Geometry: final body of the model. Coordinates: model frame, mm. A direction names the side the tool comes from. Coordinates: 2 decimals unless noted, no trailing zeros. Order: outer loops, then holes, each group sorted by start corner. A loop starts at its lowest first (then second) coordinate and runs counter-clockwise, first axis right, second up. Notation, with made-up numbers: (4, -40) - (33, -40) arc R15 cw to (33, -25) - close; hole circle Ø5 at (-26.75, 48). An arc over 180 degrees is marked (long way). Use a Markdown table: item, result. Add a question column.
```python
from build123d import *

# Parameters (mm, degrees)
SKETCH1_W           = 13
SKETCH1_H           = 17
BOSS_EXTRUDE1_DEPTH = 30
SKETCH2_R           = 5.75
CUT_EXTRUDE1_DEPTH  = 5
SKETCH3_W           = 3
SKETCH3_H           = 10
CUT_EXTRUDE2_DEPTH  = 32.851216617
SKETCH4_W           = 27
SKETCH4_H           = 17
BOSS_EXTRUDE2_DEPTH = 2
SKETCH5_W           = 7
SKETCH5_H           = 17
BOSS_EXTRUDE3_DEPTH = 20
SKETCH6_W           = 7
SKETCH6_H           = 3.5
BOSS_EXTRUDE4_DEPTH = 5
SKETCH7_R           = 2.5
CUT_EXTRUDE3_DEPTH  = 7
CUT_EXTRUDE4_DEPTH  = 42.632319176
CUT_EXTRUDE5_DEPTH  = 1
SKETCH11_W          = 0.75
SKETCH11_H          = 24
CUT_EXTRUDE6_DEPTH  = 1
SKETCH12_W          = 8
SKETCH12_H          = 0.75
CUT_EXTRUDE7_DEPTH  = 1
CUT_EXTRUDE8_DEPTH  = 13
SKETCH14_W          = 10
SKETCH14_H          = 15
CUT_EXTRUDE9_DEPTH  = 3
CHAMFER1_SIZE       = 3
BOSS_EXTRUDE5_DEPTH = 8
BOSS_EXTRUDE6_DEPTH = 1


with BuildPart() as part:
    # Sketch1 → Boss-Extrude1 (new body)
    with BuildSketch(Plane(origin=(0, 0, 0), x_dir=(1, 0, 0), z_dir=(0, 1, 0))):
        Rectangle(SKETCH1_W, SKETCH1_H)
    extrude(amount=BOSS_EXTRUDE1_DEPTH)

    # Sketch2 → Cut-Extrude1 (cut)
    with BuildSketch(Plane.ZY.offset(6.5)):
        with Locations((0, -2)):
            Circle(SKETCH2_R)
    extrude(amount=-CUT_EXTRUDE1_DEPTH, mode=Mode.SUBTRACT)

    # Sketch3 → Cut-Extrude2 (cut, through all)
    with BuildSketch(Plane.XZ):
        with Locations((5, 0)):
            Rectangle(SKETCH3_W, SKETCH3_H)
    extrude(amount=-CUT_EXTRUDE2_DEPTH, mode=Mode.SUBTRACT)

    # Sketch4 → Boss-Extrude2 (add)
    with BuildSketch(Plane(origin=(0, 30, 0), x_dir=(1, 0, 0), z_dir=(0, 1, 0))):
        with Locations((7, 0)):
            Rectangle(SKETCH4_W, SKETCH4_H)
    extrude(amount=BOSS_EXTRUDE2_DEPTH)

    # Sketch5 → Boss-Extrude3 (add)
    with BuildSketch(Plane.XZ.offset(-30)):
        with Locations((17, 0)):
            Rectangle(SKETCH5_W, SKETCH5_H)
    extrude(amount=BOSS_EXTRUDE3_DEPTH)

    # Sketch6 → Boss-Extrude4 (add)
    with BuildSketch(Plane.XZ.offset(-30)):
        with Locations((10, 6.75)):
            Rectangle(SKETCH6_W, SKETCH6_H)
        with Locations((10, -6.75)):
            Rectangle(SKETCH6_W, SKETCH6_H)
    extrude(amount=BOSS_EXTRUDE4_DEPTH)

    # Sketch7 → Cut-Extrude3 (cut)
    with BuildSketch(Plane(origin=(20.5, 0, 0), x_dir=(0, 0, -1), z_dir=(1, 0, 0))):
        with Locations((0, 27.5)):
            Circle(SKETCH7_R)
    extrude(amount=-CUT_EXTRUDE3_DEPTH, mode=Mode.SUBTRACT)

    # Sketch9 → Cut-Extrude4 (cut, through all)
    with BuildSketch(Plane.XY.offset(8.5)):
        Polygon((0, 32), (-6.5, 16), (-6.5, 32), align=None)
    extrude(amount=-CUT_EXTRUDE4_DEPTH, mode=Mode.SUBTRACT)

    # Sketch10 → Cut-Extrude5 (cut)
    with BuildSketch(Plane.XZ):
        Polygon((-5.75, 5.390964663), (-5.75, 7.75), (6.5, 7.75), (6.5, 8.5), (-6.5, 8.5), (-6.5, 5.390964663), align=None)
        Polygon((-5.75, -7.75), (-5.75, -5.390964663), (-6.5, -5.390964663), (-6.5, -8.5), (6.5, -8.5), (6.5, -7.75), align=None)
    extrude(amount=-CUT_EXTRUDE5_DEPTH, mode=Mode.SUBTRACT)

    # Sketch11 → Cut-Extrude6 (cut)
    with BuildSketch(Plane(origin=(6.5, 0, 0), x_dir=(0, 0, -1), z_dir=(1, 0, 0))):
        with Locations((-8.125, 13)):
            Rectangle(SKETCH11_W, SKETCH11_H)
        with Locations((8.125, 13)):
            Rectangle(SKETCH11_W, SKETCH11_H)
    extrude(amount=-CUT_EXTRUDE6_DEPTH, mode=Mode.SUBTRACT)

    # Sketch12 → Cut-Extrude7 (cut)
    with BuildSketch(Plane.XZ.offset(-25)):
        with Locations((9.5, -8.125)):
            Rectangle(SKETCH12_W, SKETCH12_H)
        with Locations((9.5, 8.125)):
            Rectangle(SKETCH12_W, SKETCH12_H)
    extrude(amount=-CUT_EXTRUDE7_DEPTH, mode=Mode.SUBTRACT)

    # Sketch13 → Cut-Extrude8 (cut)
    with BuildSketch(Plane.XZ.offset(-10)):
        with BuildLine():
            Line((13.5, -8.5), (13.5, 8.5))
            add(Edge.make_bspline(
                [(13.5, -8.5), (15.857076701, -7.146482538), (17.987215619, 0.415145569), (16.168492061, 6.316191401), (13.5, 8.5)],
                knots=[0, 0, 0, 0, 0.5, 1, 1, 1, 1], degree=3))
        make_face()
    extrude(amount=-CUT_EXTRUDE8_DEPTH, mode=Mode.SUBTRACT)

    # Sketch14 → Cut-Extrude9 (cut)
    with BuildSketch(Plane(origin=(3.5, 0, 0), x_dir=(0, 0, -1), z_dir=(1, 0, 0))):
        with Locations((0, 22.5)):
            Rectangle(SKETCH14_W, SKETCH14_H)
    extrude(amount=-CUT_EXTRUDE9_DEPTH, mode=Mode.SUBTRACT)

    # Chamfer1
    chamfer1_edges = [part.edges().sort_by_distance(p)[0] for p in [
        (3.5, 15, 0),
    ]]
    chamfer(chamfer1_edges, length=CHAMFER1_SIZE - 0.0001)  # a hair under: the kernel refuses the full size

    # Sketch15 → Boss-Extrude5 (add)
    with BuildSketch(Plane.ZY.offset(6.5)):
        with BuildLine():
            Line((-7.322463691, 1), (-6.32455532, 1))
            ThreePointArc((-6.32455532, 1), (0, 5), (6.32455532, 1))
            Line((6.32455532, 1), (7.322463691, 1))
            ThreePointArc((7.322463691, 1), (0, 5.913183588), (-7.322463691, 1))
        make_face()
    extrude(amount=BOSS_EXTRUDE5_DEPTH)

    # Sketch16 → Boss-Extrude6 (add)
    with BuildSketch(Plane.ZY.offset(14.5)):
        with BuildLine():
            Line((-7.322463691, 1), (7.322463691, 1))
            ThreePointArc((7.322463691, 1), (0, 5.913183588), (-7.322463691, 1))
        make_face()
    extrude(amount=BOSS_EXTRUDE6_DEPTH)


solid = part.part
```
1) Section C-C (y = 5.5). Return loops of the section in (x, z), then the cut area to 3 significant figures.
2) Section B-B (y = 9). Return loops of the section in (x, z).
3) Set-up query: faces 1 (the face through (-5.75, 0.5, 6.6)), 2 (the face through (-1.5, 1, 0)), 3 (the face through (19, 10, 0)), 4 (the face through (-5.75, 0.5, -6.6)), 5 (the face through (0.5, 23, 0)). Return all of +Z, -Z, +X, -X, +Y, -Y with unobstructed straight access to the full face (end or side cutting, diameter ignored); none if empty.
4) Draft query along Z for faces 6 (the face through (2, 13.5, 0.1)), 7 (the face through (4, 17, -8.5)), 8 (the face through (20.5, 21, 0)). Return one class per face: pulls with the +Z half, pulls with the -Z half, needs draft (parallel to the pull), parting line crosses it, or undercut.
5) Section D-D (x = -7). Return loops of the section in (y, z).
6) Ray query, line 1 along Z through (x, y) = (11.5, 29); line 2 along Y through (x, z) = (16.25, 0); line 3 along Z through (x, y) = (15.25, 27.5). Return the intervals inside material, ascending.
7) Pin query (flat end, axial travel): pin 1 (4.5 mm diameter, centred on y = 11.5, z = 3, fed in from -X); pin 2 (0.8 mm diameter, centred on x = 10, z = -8.5, fed in from -Y); pin 3 (4.5 mm diameter, centred on y = 2.5, z = 1.5, fed in from +X). Return the tip coordinate at first contact, or that it passes through.
8) Section A-A (x = 9). Return loops of the section in (y, z).
Values follow:
| question | item | result |
|---|---|---|
| 1 | outline | (-15.5, -2.52) - (-6.5, -2.52) - (-6.5, -8.5) - (5.5, -8.5) - (5.5, -7.75) - (6.5, -7.75) - (6.5, -5) - (3.5, -5) - (3.5, 5) - (6.5, 5) - (6.5, 7.75) - (5.5, 7.75) - (5.5, 8.5) - (-6.5, 8.5) - (-6.5, 2.52) - (-15.5, 2.52) - close |
| 1 | area | 235 mm² |
| 2 | outline | (-6.5, -8.5) - (5.5, -8.5) - (5.5, -7.75) - (6.5, -7.75) - (6.5, -5) - (3.5, -5) - (3.5, 5) - (6.5, 5) - (6.5, 7.75) - (5.5, 7.75) - (5.5, 8.5) - (-6.5, 8.5) - close |
| 3 | face 1 | +Z, -X, -Y |
| 3 | face 2 | -Y |
| 3 | face 3 | +Z, -Z, +X, -Y |
| 3 | face 4 | -Z, -X, -Y |
| 3 | face 5 | none |
| 4 | face 6 | undercut |
| 4 | face 7 | pulls with the -Z half |
| 4 | face 8 | needs draft |
| 5 | outline | (1, -7.32) arc R7.91 ccw to (1, 7.32) - (1, 6.32) arc R7 cw to (1, -6.32) - close |
| 6 | line 1 | z = -8.5 to -5, 5 to 8.5 |
| 6 | line 2 | y = 23 to 25, 30 to 32 |
| 6 | line 3 | z = -8.5 to -2.5, 2.5 to 8.5 |
| 7 | pin 1 | stops at x = -6.5 |
| 7 | pin 2 | stops at y = 26 |
| 7 | pin 3 | stops at x = 3.5 |
| 8 | outline | (25, -7.75) - (26, -7.75) - (26, -8.5) - (32, -8.5) - (32, 8.5) - (26, 8.5) - (26, 7.75) - (25, 7.75) - (25, 5) - (30, 5) - (30, -5) - (25, -5) - close |
